Could you check a few things on this model? Use its own coordinates, in mm. Face numbers are marked on the shaded views. A direction names the side the tool comes from. Give positions to 0.01 mm unless a question says otherwise; leave off trailing zeros. Loops run counter-clockwise (first coordinate to the right, second up) from the corner with the lowest first, then second, coordinate; pieces in that order, holes last. Notation, with made-up numbers: (46.5, 0.25) -> (73.5, 0.25) arc R5 cw to (73.5, 8.25) -> close; hole circle Ø1 at (78, 60.5). An arc over 180 degrees is marked (long way). Write each question's results on one line, items separated by ' | '. Start each with the question number.
Q1. Which directions (+Z, -Z, +X, -X, +Y, -Y) give clear straight access to the entire face, cutting with the end or side of a thin tool? Please do the marked faces 5, 6 and 7.
Q2. If we section it at C-C, the plane x = -180: Give the number of separate pieces and of enclosed holes in the cut face, plus the area to 3 significant figures.
Q3. If I drill on line 1 along Z through (x, y) = (119.5, 42.5); line 2 along Z through (x, y) = (-135.5, 67); line 3 along X through (y, z) = (85, 104), over which ranges is the centre line in solid material (lowest first)?
Q4. If we section it at B-B, the plane z = -297: List the corners of the cut face in (x, y) for me.
Q5. Will these pins go through, and if not, where does the flat tip stop? P1, Ø4.5, axis at x = -224, y = 58.5, coming from the +Z side; P2, Ø4.5, axis at x = 174, y = 52, coming from the -Z side; P3, Ø6, axis at y = 9, z = -325, coming from the -X side; P4, Ø3, axis at x = -31.5, z = -103.5, coming from the -Y side.
Q6. We'd pull the mould along X, two halves only. Please class the marked faces 1, 2, 3 and 4: released by +X, released by -X, zero draft, split by the parting line, or undercut.
Q7. If we section it at A-A, the plane x = -19.5: List the corners of the cut face in (y, z) for me.
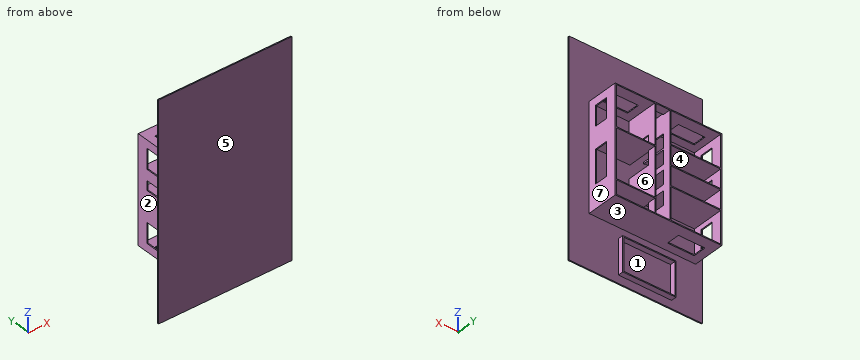
Autodesk Inventor part; units mm, degrees
ref_plane "Plano de trabajo1" through (-225, 4, 200) normal (0, 0, 1) x (1, 0, 0)
ref_plane "Plano de trabajo2" through (-30, 4, 200) normal (1, 0, 0) x (0, 0, -1)
ref_plane "YZ Plane" through (0, 0, 0) normal (1, 0, 0) x (0, 1, 0)
sketch "Boceto1" plane through (0, 0, 0) normal (0, 1, 0) x (-1, 0, 0)
  line L0 (-250, 400) -> (250, 400)
  line L1 (250, 400) -> (250, -400)
  line L2 (250, -400) -> (-250, -400)
  line L3 (-250, -400) -> (-250, 400)
  line L4 (-250, 400) -> (250, -400) construction
  line L5 (250, 400) -> (-250, -400) construction
  line L6 (-175, 200) -> (225, 200)
  line L7 (225, 200) -> (225, -200)
  line L8 (225, -200) -> (-175, -200)
  line L9 (-175, -200) -> (-175, 200)
  line L10 (-175, 200) -> (225, -200) construction
  line L11 (225, 200) -> (-175, -200) construction
  point P0 (0, 0)
  point P1 (25, 0)
  dimension "d0" = 500
  dimension "d1" = 800
  dimension "d4" = 400
  dimension "d5" = 400
  dimension "d6" = 200
  dimension "d7" = 75
extrude "Extrusión1" add sketch "Boceto1" along normal blind 4 contours L0 L1 L2 L3 | L6 L7 L8 L9
sketch "Boceto2" plane through (0, 4, 0) normal (0, 1, 0) x (1, 0, 0)
  line L0 (175, -200) -> (-225, -200)
  line L1 (-225, -200) -> (-225, 200)
  line L2 (-225, 200) -> (175, 200)
  line L3 (175, 200) -> (175, -200)
  line L4 (175, -200) -> (-225, 200) construction
  line L5 (-225, -200) -> (175, 200) construction
  line L6 (250, -400) -> (250, 400)
  line L7 (250, 400) -> (-250, 400)
  line L8 (-221, -196) -> (-34, -196)
  line L9 (-34, -196) -> (-34, -76)
  line L10 (-34, -76) -> (-221, -76)
  line L11 (-221, -76) -> (-221, -196)
  line L12 (171, -196) -> (26, -196)
  line L13 (26, -196) -> (26, -46)
  line L14 (26, -46) -> (171, -46)
  line L15 (171, -46) -> (171, -196)
  line L16 (171, 196) -> (26, 196)
  line L17 (26, 196) -> (26, -42)
  line L18 (26, -42) -> (171, -42)
  line L19 (171, -42) -> (171, 196)
  line L20 (-34, -72) -> (-221, -72)
  line L21 (-221, -72) -> (-221, 72)
  line L22 (-221, 72) -> (-34, 72)
  line L23 (-34, 72) -> (-34, -72)
  line L24 (-34, 76) -> (-221, 76)
  line L25 (-221, 76) -> (-221, 196)
  line L26 (-221, 196) -> (-34, 196)
  line L27 (-34, 196) -> (-34, 76)
  line L28 (-30, 196) -> (22, 196)
  line L29 (22, 196) -> (22, 122)
  line L30 (-30, 122) -> (-30, 196)
  line L31 (-34, 0) -> (-34, -2)
  line L32 (-34, -2) -> (-34, 2)
  line L33 (-34, 2) -> (-221, 2)
  line L34 (-221, -2) -> (-34, -2)
  line L35 (-30, -200) -> (-30, 122)
  line L36 (22, 122) -> (22, -200)
  line L37 (-30, -196) -> (22, -196)
  line L38 (26, 196) -> (26, 144)
  line L39 (26, 144) -> (26, 140)
  line L40 (26, 140) -> (171, 140)
  line L41 (171, 144) -> (26, 144)
  point P0 (0, 0)
  point P1 (-25, 0)
  point P2 (-30, 126)
  point P3 (22, 126)
  dimension "d8" = 400
  dimension "d9" = 400
  dimension "d10" = 75
  dimension "d11" = 200
  dimension "d12" = 4
  dimension "d13" = 4
  dimension "d14" = 4
  dimension "d15" = 4
  dimension "d16" = 4
  dimension "d17" = 60
  dimension "d18" = 145
  dimension "d19" = 150
  dimension "d20" = 120
  dimension "d21" = 120
  dimension "d22" = 4
  dimension "d23" = 4
  dimension "d24" = 2
  dimension "d25" = 4
  dimension "d27" = 4
  dimension "d39" = 52
  dimension "d40" = 4
ref_plane "Plano de trabajo1" through (-225, 4, 200) normal (0, 0, 1) x (1, 0, 0)
sketch "Boceto3" plane through (-225, 4, 200) normal (0, 0, 1) x (1, 0, 0)
  line L0 (195, 0) -> (195, 120)
  line L1 (247, 0) -> (247, 120)
  line L2 (195, 0) -> (247, 0)
  line L3 (247, 0) -> (247, 90)
  line L4 (247, 90) -> (195, 90)
  line L5 (195, 90) -> (195, 0)
  point P0 (225, -4)
  dimension "d31" = 90
extrude "Extrusión3" cut sketch "Boceto3" against normal blind 120
ref_plane "Plano de trabajo2" through (-30, 4, 200) normal (1, 0, 0) x (0, 0, -1)
sketch "Boceto4" plane through (-30, 4, 200) normal (1, 0, 0) x (0, 0, -1)
  line L0 (124, 0) -> (124, 120)
  line L1 (124, 0) -> (72, 0)
  line L2 (72, 0) -> (72, 90)
  line L3 (72, 90) -> (124, 90)
  line L4 (124, 90) -> (124, 0)
  line L5 (0, 0) -> (400, 0)
  line L6 (129.886, 90) -> (181.886, 90)
  line L7 (181.886, 90) -> (181.886, 0)
  line L8 (181.886, 0) -> (129.886, 0)
  line L9 (129.886, 0) -> (129.886, 90)
  line L10 (202, 0) -> (202, 120)
  line L11 (202, 0) -> (254, 0)
  line L12 (254, 0) -> (254, 90)
  line L13 (254, 90) -> (202, 90)
  line L14 (202, 90) -> (202, 0)
  line L15 (276, 0) -> (276, 120)
  line L16 (396, 0) -> (276, 0)
  line L17 (276, 90) -> (328, 90)
  line L18 (328, 90) -> (328, 0)
  line L19 (328, 0) -> (276, 0)
  line L20 (276, 0) -> (276, 90)
  point P0 (200, -4)
  dimension "d34" = 52
  dimension "d35" = 90
  dimension "d36" = 52
  dimension "d37" = 52
  dimension "d38" = 52
extrude "Extrusión4" add sketch "Boceto2" along normal blind 120 contours L0 L36 L29 L28 L30 L35 L1 L2 L3 | L0 L35 L37 L36 | L19 L40 L17 L41 | L34 L21 L33 L23
extrude "Extrusión5" cut sketch "Boceto4" against normal blind 120
sketch "Boceto5" plane through (22, 4, -196) normal (-1, 0, 0) x (0, 0, 1)
  line L0 (596, 0) -> (-204, 0)
  line L1 (0, 0) -> (52, 0)
  line L2 (52, 0) -> (52, 90)
  line L3 (52, 90) -> (0, 90)
  line L4 (0, 90) -> (0, 0)
  line L5 (238, 0) -> (238, 120)
  line L6 (238, 90) -> (186, 90)
  line L7 (186, 90) -> (186, 0)
  line L8 (186, 0) -> (238, 0)
  line L9 (238, 0) -> (238, 90)
  line L10 (242, 0) -> (242, 120)
  line L11 (242, 0) -> (392, 0)
  line L12 (242, 90) -> (294, 90)
  line L13 (294, 90) -> (294, 0)
  line L14 (294, 0) -> (242, 0)
  line L15 (242, 0) -> (242, 90)
  line L16 (0, 0) -> (0, 120)
  point P0 (196, -4)
  dimension "d45" = 52
  dimension "d46" = 90
  dimension "d47" = 52
  dimension "d48" = 52
  dimension "d108" = 0
extrude "Extrusión6" cut sketch "Boceto5" against normal blind 120
sketch "Boceto6" plane through (-225, 4, 200) normal (0, 0, 1) x (1, 0, 0)
  line L0 (195, 0) -> (247, 0)
  line L1 (247, 0) -> (247, 120)
  line L2 (195, 0) -> (247, 0)
  line L3 (247, 0) -> (247, 90)
  line L4 (247, 90) -> (195, 90)
  line L5 (195, 90) -> (195, 0)
  point P0 (225, -4)
  dimension "d51" = 90
extrude "Extrusión7" cut sketch "Boceto6" against normal blind 120
sketch "Boceto7" plane through (0, 4, 0) normal (0, 1, 0) x (1, 0, 0)
  line L0 (-135, 240) -> (65, 240)
  line L1 (65, 240) -> (65, 370)
  line L2 (65, 370) -> (-135, 370)
  line L3 (-135, 370) -> (-135, 240)
  line L4 (175, 200) -> (-225, 200)
  line L5 (-250, 400) -> (-250, -400)
  line L6 (61, 244) -> (-131, 244)
  line L7 (-131, 244) -> (-131, 366)
  line L8 (-131, 366) -> (61, 366)
  line L9 (61, 366) -> (61, 244)
  line L10 (61, 244) -> (-131, 366) construction
  line L11 (-131, 244) -> (61, 366) construction
  point P0 (0, 0)
  point P1 (-35, 305)
  dimension "d54" = 200
  dimension "d55" = 130
  dimension "d56" = 40
  dimension "d57" = 115
  dimension "d58" = 192
  dimension "d59" = 122
  dimension "d60" = 4
  dimension "d61" = 4
extrude "Extrusión8" add sketch "Boceto7" along normal blind 20
sketch "Boceto8" plane through (-225, 4, 200) normal (0, 0, 1) x (1, 0, 0)
  line L0 (30, 30) -> (130, 30)
  line L1 (130, 30) -> (130, 80)
  line L2 (130, 80) -> (30, 80)
  line L3 (30, 80) -> (30, 30)
  line L4 (30, 30) -> (130, 80) construction
  line L5 (130, 30) -> (30, 80) construction
  line L6 (195, 0) -> (0, 0)
  line L7 (0, 0) -> (0, 120)
  point P0 (225, -4)
  point P1 (80, 55)
  dimension "d64" = 100
  dimension "d65" = 50
  dimension "d66" = 30
  dimension "d67" = 30
extrude "Extrusión9" cut sketch "Boceto8" against normal blind 10
sketch "Boceto9" plane through (-225, 4, -200) normal (-1, 0, 0) x (0, 0, 1)
  line L0 (295, 30) -> (370, 30)
  line L1 (370, 30) -> (370, 80)
  line L2 (370, 80) -> (295, 80)
  line L3 (295, 80) -> (295, 30)
  line L4 (295, 30) -> (370, 80) construction
  line L5 (370, 30) -> (295, 80) construction
  line L6 (400, 0) -> (400, 120)
  line L7 (400, 0) -> (0, 0)
  point P0 (200, -4)
  point P1 (332.5, 55)
  dimension "d70" = 75
  dimension "d71" = 50
  dimension "d72" = 30
  dimension "d73" = 30
extrude "Extrusión10" cut sketch "Boceto9" against normal blind 10
sketch "Boceto10" plane through (-225, 4, -200) normal (-1, 0, 0) x (0, 0, 1)
  line L0 (30, 30) -> (105, 30)
  line L1 (105, 30) -> (105, 80)
  line L2 (105, 80) -> (30, 80)
  line L3 (30, 80) -> (30, 30)
  line L4 (30, 30) -> (105, 80) construction
  line L5 (105, 30) -> (30, 80) construction
  line L6 (0, 0) -> (0, 120)
  line L7 (-200, 0) -> (600, 0)
  line L8 (219.5, 30) -> (254.5, 30)
  line L9 (254.5, 30) -> (254.5, 80)
  line L10 (254.5, 80) -> (219.5, 80)
  line L11 (219.5, 80) -> (219.5, 30)
  line L12 (219.5, 30) -> (254.5, 80) construction
  line L13 (254.5, 30) -> (219.5, 80) construction
  line L14 (272, 0) -> (272, 120)
  point P0 (200, -4)
  point P1 (67.5, 55)
  point P2 (237, 55)
  dimension "d76" = 75
  dimension "d77" = 50
  dimension "d78" = 30
  dimension "d79" = 30
  dimension "d80" = 35
  dimension "d81" = 50
  dimension "d82" = 30
  dimension "d83" = 17.5
extrude "Extrusión11" cut sketch "Boceto10" against normal blind 10
sketch "Boceto11" plane through (-225, 4, 200) normal (0, 0, 1) x (1, 0, 0)
  line L0 (280, 30) -> (370, 30)
  line L1 (370, 30) -> (370, 80)
  line L2 (370, 80) -> (280, 80)
  line L3 (280, 80) -> (280, 30)
  line L4 (280, 30) -> (370, 80) construction
  line L5 (370, 30) -> (280, 80) construction
  line L6 (-25, 0) -> (475, 0)
  line L7 (400, 0) -> (400, 120)
  point P0 (225, -4)
  point P1 (325, 55)
  dimension "d86" = 90
  dimension "d88" = 30
  dimension "d89" = 50
  dimension "d90" = 30
extrude "Extrusión12" cut sketch "Boceto11" against normal blind 10
sketch "Boceto12" plane through (175, 4, -200) normal (0, 0, -1) x (-1, 0, 0)
  line L0 (270, 30) -> (370, 30)
  line L1 (370, 30) -> (370, 80)
  line L2 (370, 80) -> (270, 80)
  line L3 (270, 80) -> (270, 30)
  line L4 (270, 30) -> (370, 80) construction
  line L5 (370, 30) -> (270, 80) construction
  line L6 (400, 0) -> (400, 120)
  line L7 (-75, 0) -> (425, 0)
  point P0 (175, -4)
  point P1 (320, 55)
  dimension "d93" = 100
  dimension "d94" = 50
  dimension "d95" = 30
  dimension "d96" = 30
extrude "Extrusión13" cut sketch "Boceto12" against normal blind 10
sketch "Boceto13" plane through (175, 4, 200) normal (1, 0, 0) x (0, 0, -1)
  line L0 (30, 30) -> (105, 30)
  line L1 (105, 80) -> (30, 80)
  line L2 (30, 30) -> (105, 30)
  line L3 (105, 30) -> (105, 80)
  line L4 (105, 80) -> (30, 80)
  line L5 (30, 80) -> (30, 30)
  point P0 (200, -4)
extrude "Extrusión14" cut sketch "Boceto13" against normal blind 10
sketch "Boceto14" plane through (175, 4, 200) normal (1, 0, 0) x (0, 0, -1)
  line L0 (186.5, 30) -> (311.5, 30)
  line L1 (311.5, 30) -> (311.5, 80)
  line L2 (311.5, 80) -> (186.5, 80)
  line L3 (186.5, 80) -> (186.5, 30)
  line L4 (186.5, 30) -> (311.5, 80) construction
  line L5 (311.5, 30) -> (186.5, 80) construction
  line L6 (-200, 0) -> (600, 0)
  line L7 (158, 0) -> (158, 120)
  point P0 (200, -4)
  point P1 (249, 55)
  dimension "d101" = 125
  dimension "d102" = 50
  dimension "d103" = 30
  dimension "d105" = 91
extrude "Extrusión15" cut sketch "Boceto14" against normal blind 10
properties part number "maqueta casa"
Final values:
1) face 5: +Z, -Z, +X, -X, -Y | face 6: +Y | face 7: +Z, -Z, +X, +Y
2) separate pieces: 3 | enclosed holes: 0 | area: 5,200 mm²
3) line 1: z = -200 to -196, -144 to -140, 42 to 46 | line 2: z = -76 to -72, -2 to 2, 72 to 76 | line 3: x = -225 to -221, 22 to 26, 171 to 175
4) outline: (-250, 0) -> (250, 0) -> (250, 4) -> (65, 4) -> (65, 24) -> (61, 24) -> (61, 4) -> (-131, 4) -> (-131, 24) -> (-135, 24) -> (-135, 4) -> (-250, 4) -> close
5) P1: stops at z = 200 | P2: stops at z = -200 | P3: stops at x = -135 | P4: stops at y = 0
6) face 1: undercut | face 2: released by -X | face 3: zero draft | face 4: undercut
7) outline: (0, -400) -> (4, -400) -> (4, -370) -> (24, -370) -> (24, -366) -> (4, -366) -> (4, -244) -> (24, -244) -> (24, -240) -> (4, -240) -> (4, -200) -> (124, -200) -> (124, -196) -> (4, -196) -> (4, 400) -> (0, 400) -> close; (94, 196) -> (124, 196) -> (124, 200) -> (94, 200) -> close
